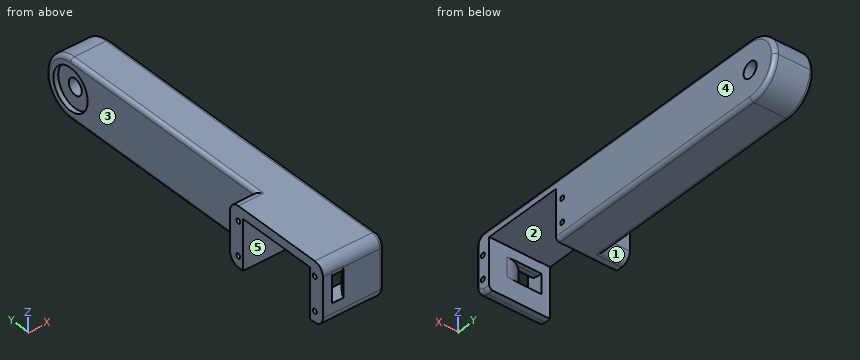
from build123d import *

# Parameters (mm, degrees)
SKETCH1_W                 = 20
SKETCH1_H                 = 30
BOSS_EXTRUDE1_DEPTH       = 183.3
SKETCH13_W                = 30
SKETCH13_H                = 57
BOSS_EXTRUDE2_DEPTH       = 11
SKETCH3_W                 = 20.6
SKETCH3_H                 = 41
CUT_EXTRUDE1_DEPTH        = 40
SKETCH11_R                = 10.5
CUT_EXTRUDE4_DEPTH        = 2.4
SKETCH12_R                = 4
CUT_EXTRUDE5_DEPTH        = 185.752943143
SKETCH14_W                = 31
SKETCH14_H                = 41
CUT_EXTRUDE6_DEPTH        = 25.3
F_2_CLEARANCE_HOLE2_D     = 2.4384
F_2_CLEARANCE_HOLE2_DEPTH = 6.35
F_2_CLEARANCE_HOLE2_TIP   = 0.732569267
CUT_EXTRUDE8_START        = -2
CUT_EXTRUDE8_DEPTH        = 1.6
F_2_CLEARANCE_HOLE3_D     = 2.4384
F_2_CLEARANCE_HOLE3_DEPTH = 6.35
F_2_CLEARANCE_HOLE3_TIP   = 1.2192
FILLET3_R                 = 15
FILLET4_R                 = 5
FILLET5_R                 = 2
SKETCH21_W                = 6
SKETCH21_H                = 10
CUT_EXTRUDE9_DEPTH        = 8
FILLET6_R                 = 12
FILLET7_R                 = 6
CUT_EXTRUDE10_START       = -2
CUT_EXTRUDE10_DEPTH       = 1.8


# Some blends are built 0.0001 mm under size
with BuildPart() as part:
    # Sketch1 → Boss-Extrude1 (new body)
    with BuildSketch(Plane(origin=(0, 0, 0), x_dir=(1, 0, 0), z_dir=(0, 1, 0))):
        Rectangle(SKETCH1_W, SKETCH1_H)
    extrude(amount=BOSS_EXTRUDE1_DEPTH)

    # Sketch13 → Boss-Extrude2 (add)
    with BuildSketch(Plane.ZY.offset(10)):
        with Locations((0, 28.5)):
            Rectangle(SKETCH13_W, SKETCH13_H)
    extrude(amount=BOSS_EXTRUDE2_DEPTH)

    # Sketch3 → Cut-Extrude1 (cut)
    with BuildSketch(Plane(origin=(10, 0, 0), x_dir=(0, 0, -1), z_dir=(1, 0, 0))):
        with Locations((0, 28.5)):
            Rectangle(SKETCH3_W, SKETCH3_H)
    extrude(amount=-CUT_EXTRUDE1_DEPTH, mode=Mode.SUBTRACT)

    # Sketch11 → Cut-Extrude4 (cut)
    with BuildSketch(Plane.ZY.offset(10)):
        with Locations((0, 168.3)):
            Circle(SKETCH11_R)
    extrude(amount=-CUT_EXTRUDE4_DEPTH, mode=Mode.SUBTRACT)

    # Sketch12 → Cut-Extrude5 (cut, through all)
    with BuildSketch(Plane.ZY.offset(7.6)):
        with Locations((0, 168.3)):
            Circle(SKETCH12_R)
    extrude(amount=-CUT_EXTRUDE5_DEPTH, mode=Mode.SUBTRACT)

    # Sketch14 → Cut-Extrude6 (cut)
    with BuildSketch(Plane(origin=(0, 0, -15), x_dir=(-1, 0, 0), z_dir=(0, 0, -1))):
        with Locations((5.5, 28.5)):
            Rectangle(SKETCH14_W, SKETCH14_H)
    extrude(amount=-CUT_EXTRUDE6_DEPTH, mode=Mode.SUBTRACT)

    # #2 Clearance Hole2
    with Locations(Plane.ZY.offset(21)):
        with Locations((-9.5, 5), (7.5, 5), (-9.5, 52), (7.5, 52)):
            Hole(F_2_CLEARANCE_HOLE2_D / 2, depth=F_2_CLEARANCE_HOLE2_DEPTH)
            with Locations((0, 0, -(F_2_CLEARANCE_HOLE2_DEPTH + F_2_CLEARANCE_HOLE2_TIP / 2))):  # 118° drill point
                Cone(0, F_2_CLEARANCE_HOLE2_D / 2, F_2_CLEARANCE_HOLE2_TIP, mode=Mode.SUBTRACT)

    # Sketch18 → Cut-Extrude8 (cut)
    with BuildSketch(Plane.ZY.offset(21).offset(CUT_EXTRUDE8_START)):
        Polygon((-12.329016319, 5), (-10.91450816, 2.55), (-8.08549184, 2.55), (-6.670983681, 5), (-8.08549184, 7.45), (-10.91450816, 7.45), align=None)
        Polygon((10.329016319, 5), (8.91450816, 7.45), (6.08549184, 7.45), (4.670983681, 5), (6.08549184, 2.55), (8.91450816, 2.55), align=None)
        Polygon((4.670983681, 52), (6.08549184, 49.55), (8.91450816, 49.55), (10.329016319, 52), (8.91450816, 54.45), (6.08549184, 54.45), align=None)
        Polygon((-6.670983681, 52), (-8.08549184, 54.45), (-10.91450816, 54.45), (-12.329016319, 52), (-10.91450816, 49.55), (-8.08549184, 49.55), align=None)
    extrude(amount=-CUT_EXTRUDE8_DEPTH, mode=Mode.SUBTRACT)

    # #2 Clearance Hole3
    with Locations(Plane(origin=(10, 0, 0), x_dir=(0, 0, -1), z_dir=(1, 0, 0))):
        with Locations((8.22, 4.1), (-3.52, 4.1), (-3.52, 52.9), (8.22, 52.9)):
            Hole(F_2_CLEARANCE_HOLE3_D / 2, depth=F_2_CLEARANCE_HOLE3_DEPTH)
            with Locations((0, 0, -(F_2_CLEARANCE_HOLE3_DEPTH + F_2_CLEARANCE_HOLE3_TIP / 2))):  # 90° drill point
                Cone(0, F_2_CLEARANCE_HOLE3_D / 2, F_2_CLEARANCE_HOLE3_TIP, mode=Mode.SUBTRACT)

    # Fillet3
    fillet3_edges = [part.edges().sort_by_distance(p)[0] for p in [
        (0, 183.3, -15),
        (0, 183.3, 15),
    ]]
    fillet(fillet3_edges, radius=FILLET3_R - 0.0001)  # a hair under: the kernel refuses the full size

    # Fillet4
    fillet4_edges = [part.edges().sort_by_distance(p)[0] for p in [
        (-15.5, 57, -15),
        (-15.5, 57, 15),
        (-5.5, 0, -15),
        (-5.5, 0, 15),
    ]]
    fillet(fillet4_edges, radius=FILLET4_R)

    # Fillet5
    fillet5_edges = [part.edges().sort_by_distance(p)[0] for p in [
        (-10, 110.15005, 15),
        (-10, 110.15005, -15),
        (-10, 178.906631007, 10.606631007),
        (-10, 178.906631007, -10.606631007),
        (10, 108.65005, -15),
        (10, 86.65005, 15),
        (10, 178.906631007, 10.606631007),
        (10, 178.906631007, -10.606631007),
        (10, 0, 0),
        (10, 1.464466094, 13.535533906),
        (10, 1.464466094, -13.535533906),
        (10, 6.5, -15),
    ]]
    fillet(fillet5_edges, radius=FILLET5_R)

    # Sketch21 → Cut-Extrude9 (cut)
    with BuildSketch(Plane.XZ):
        with Locations((-13.5, 0)):
            Rectangle(SKETCH21_W, SKETCH21_H)
    extrude(amount=-CUT_EXTRUDE9_DEPTH, mode=Mode.SUBTRACT)

    # Fillet6
    # the kernel refuses this fillet: 12 mm, written as the material it takes off along each edge
    with BuildSketch(Plane(origin=(-10.5, 8, -5), x_dir=(1, 0, 0), z_dir=(0, 0, 1))) as fillet6_piece_1:
        with BuildLine():
            CenterArc((11.313708499, -12), FILLET6_R, 90, 70.528779366)
            Line((0, -8), (0, 0))
            Line((0, 0), (11.313708499, 0))
        make_face()
    extrude(amount=10, mode=Mode.SUBTRACT)

    # Fillet7
    # the kernel refuses this fillet: 6 mm, written as the material it takes off along each edge
    with BuildSketch(Plane(origin=(4.5, 0, 5), x_dir=(0, 1, 0), z_dir=(-1, 0, 0))) as fillet7_piece_1_section:
        with BuildLine():
            CenterArc((FILLET7_R, -FILLET7_R), FILLET7_R, 90, 90)
            Line((0, -FILLET7_R), (0, 0))
            Line((0, 0), (FILLET7_R, 0))
        make_face()
    fillet7_piece_1 = extrude(amount=21, mode=Mode.PRIVATE)
    fillet7_piece_1 = fillet7_piece_1 - Plane(origin=(0.813708499, -4, 5), x_dir=(1, 0, 0), z_dir=(0, 0, -1)) * Cylinder(12, 66, mode=Mode.PRIVATE)
    add(fillet7_piece_1, mode=Mode.SUBTRACT)

    # Sketch22 → Cut-Extrude10 (cut)
    with BuildSketch(Plane(origin=(10, 0, 0), x_dir=(0, 0, -1), z_dir=(1, 0, 0)).offset(CUT_EXTRUDE10_START)):
        Polygon((-6.349016319, 52.9), (-4.93450816, 50.45), (-2.10549184, 50.45), (-0.690983681, 52.9), (-2.10549184, 55.35), (-4.93450816, 55.35), align=None)
        Polygon((5.390983681, 52.9), (6.80549184, 50.45), (9.63450816, 50.45), (11.049016319, 52.9), (9.63450816, 55.35), (6.80549184, 55.35), align=None)
        Polygon((-6.349016319, 4.1), (-4.93450816, 1.65), (-2.10549184, 1.65), (-0.690983681, 4.1), (-2.10549184, 6.55), (-4.93450816, 6.55), align=None)
        Polygon((5.390983681, 4.1), (6.80549184, 1.65), (9.63450816, 1.65), (11.049016319, 4.1), (9.63450816, 6.55), (6.80549184, 6.55), align=None)
    extrude(amount=-CUT_EXTRUDE10_DEPTH, mode=Mode.SUBTRACT)


solid = part.part
The listing builds one solid part. Answer for the finished solid, in the listing's coordinates (mm). Face numbers are marked on the shaded views. A direction names the side the tool comes from. Coordinates: 2 decimals unless noted, no trailing zeros. Order: outer loops, then holes, each group sorted by start corner. A loop starts at its lowest first (then second) coordinate and runs counter-clockwise, first axis right, second up. Notation, with made-up numbers: (-29, 88) -> (9, 88) arc R11 ccw to (9, 98) -> close; hole circle Ø4 at (3.5, -38). An arc over 180 degrees is marked (long way). Answer in a Markdown table with one row per item. Add a question column.
Item 1: Which of the six approach directions +Z, -Z, +X, -X, +Y, -Y give full straight-line access (tool end or side, diameter ignored) to the marked faces 4 and 5?
Item 2: Find section A-A (y = 83). Write down the section's boundary in (x, z).
Item 3: Find the intervals of material crossed by L1, parallel to Z at x = -16.35, y = 52; L2, parallel to Y at x = -20.05, z = 7.5; L3, parallel to Y at x = -9.4, z = 0, in increasing order. Write a range as from..to.
Item 4: Find section C-C (y = 15). Write down the section's boundary in (x, z).
Item 5: Each of these flat-tipped pins is pushed along its axis until it touches: P1, Ø2, axis at y = 5, z = -9.5, coming from the -X side; P2, Ø2, axis at y = 141.5, z = -8, coming from the -X side; P3, Ø4, axis at x = -14, z = 10.5, coming from the +Y side; P4, Ø6, axis at y = 20, z = 6, coming from the -X side. Where does it stop, or does it pass through?
Item 6: Determine the mould class of the marked faces 1, 2 and 3 for opening direction Y: +Y half, -Y half, draft (parallel to the pull), parting line (faces both ways), or undercut.
Result set:
| question | item | result |
|---|---|---|
| 1 | face 4 | +Z, -Z, +X, +Y, -Y |
| 1 | face 5 | -Z, +X, -X |
| 2 | outline | (-10, -13) arc R2 ccw to (-8, -15) -> (8, -15) arc R2 ccw to (10, -13) -> (10, 13) arc R2 ccw to (8, 15) -> (-8, 15) arc R2 ccw to (-10, 13) -> close |
| 3 | L1 | z = -15..-10.72, -8.28..6.28, 8.72..15 |
| 3 | L2 | y = 0..3.78, 6.22..8, 49..50.78, 53.22..57 |
| 3 | L3 | y = 0..2.3, 49..157.8, 178.8..182.73 |
| 4 | outline | (-21, 10.3) -> (10, 10.3) -> (10, 13) arc R2 ccw to (8, 15) -> (-21, 15) -> close |
| 5 | P1 | stops at x = -14.52 |
| 5 | P2 | stops at x = -10 |
| 5 | P3 | stops at y = 57 |
| 5 | P4 | passes through |
| 6 | face 1 | +Y half |
| 6 | face 2 | undercut |
| 6 | face 3 | draft |
